```python
from build123d import *

# Parameters (mm, degrees)
SKETCH1_R           = 11
BOSS_EXTRUDE1_DEPTH = 8
SKETCH2_R           = 3
CUT_EXTRUDE1_DEPTH  = 7
FILLET1_R           = 1


with BuildPart() as part:
    # Sketch1 → Boss-Extrude1 (new body)
    with BuildSketch(Plane(origin=(0, 0, 0), x_dir=(0, 0, -1), z_dir=(1, 0, 0))):
        Circle(SKETCH1_R)
    extrude(amount=BOSS_EXTRUDE1_DEPTH)

    # Sketch2 → Cut-Extrude1 (cut)
    with BuildSketch(Plane.ZY):
        Circle(SKETCH2_R)
    extrude(amount=-CUT_EXTRUDE1_DEPTH, mode=Mode.SUBTRACT)

    # Fillet1
    fillet1_edges = [part.edges().sort_by_distance(p)[0] for p in [
        (8, 0, 11),
    ]]
    fillet(fillet1_edges, radius=FILLET1_R)


solid = part.part
```
Work out the finished part from the listing and answer in its coordinate system (mm). A direction names the side the tool comes from. Give positions to 0.01 mm unless a question says otherwise; leave off trailing zeros. Order: outer loops, then holes, each group sorted by start corner. A loop starts at its lowest first (then second) coordinate and runs counter-clockwise, first axis right, second up.
1. Section C-C, the plane x = 3 is taken. Determine the outline of the cut face in (y, z), and give its area (3 significant figures).
Result sheet:
outline: circle Ø22 at (0, 0); hole circle Ø6 at (0, 0)
area: 352 mm2
2. For faces 1 (the flat face through (0, -2.3, -2.3)), 2 (the cylindrical face through (3, 0, -3)), determine the directions among +Z, -Z, +X, -X, +Y, -Y from which every point of the face is accessible in a straight line to the end or side of a thin tool.
Result sheet:
face 1: +Z, -Z, -X, +Y, -Y
face 2: -X
3. Section A-A, the plane z = 0 is taken. Determine the outline of the cut face in (x, y).
Result sheet:
outline: (0, -11) - (7, -11) arc R1 ccw to (8, -10) - (8, 10) arc R1 ccw to (7, 11) - (0, 11) - (0, 3) - (7, 3) - (7, -3) - (0, -3) - close
4. Straight lines are drawn through the part: L1, parallel to Y at x = 1.5, z = 0; L2, parallel to X at y = 2.75, z = -1; L3, parallel to Z at x = 6.75, y = 2. For each, find the intervals that lie inside material, in ascending order.
Result sheet:
L1: y = -11 to -3, 3 to 11
L2: x = 7 to 8
L3: z = -10.82 to -2.24, 2.24 to 10.82
5. Each of these flat-tipped pins is pushed along its axis until it touches: P1, Ø1.5, axis at x = 2, z = 8.5, coming from the -Y side; P2, Ø3, axis at y = -1, z = -1, coming from the -X side; P3, Ø2, axis at x = 3.5, z = 5.5, coming from the +Y side. Where does it stop, or does it pass through?
Result sheet:
P1: stops at y = -7.81
P2: stops at x = 7
P3: stops at y = 10.04
6. The mould has two halves that part along Z. Classify faces 3 (the cylindrical face through (3.45, -10.74, 2.38)), 4 (the flat face through (7, 0, 0)), 5 (the flat face through (8, 0, 0)): released by +Z, released by -Z, zero draft, split by the parting line, or undercut.
Result sheet:
face 3: split by the parting line
face 4: undercut
face 5: zero draft
